```python
from build123d import *

# Parameters (mm, degrees)
SKETCH1_R                     = 14.605
BOSS_EXTRUDE2_DEPTH           = 25.4
SKETCH10_R                    = 5.715
CUT_EXTRUDE5_DEPTH            = 48.424233935
SKETCH11_R                    = 6.6675
CUT_EXTRUDE6_DEPTH            = 1.27
SKETCH12_OUTSIDE_W            = 40.908
SKETCH12_OUTSIDE_H            = 40.908
SKETCH12_OUTSIDE_R            = 10.414
CUT_EXTRUDE7_DEPTH            = 17.78
CIRPATTERN1_COUNT             = 3
CIRPATTERN2_COUNT             = 2
SKETCH26_R                    = 1.651
CUT_EXTRUDE8_DEPTH            = 8.89
CIRPATTERN3_COUNT             = 2
SKETCH27_R                    = 0.79375
CUT_EXTRUDE9_DEPTH            = 24.13
TAP_DRILL_FOR_0_80_TAP3_D     = 1.19126
TAP_DRILL_FOR_0_80_TAP3_DEPTH = 6.35
TAP_DRILL_FOR_0_80_TAP3_TIP   = 0.499792913
TAP_DRILL_FOR_2_56_TAP1_D     = 1.778
CIRPATTERN4_COUNT             = 2


with BuildPart() as part:
    # Sketch1 → Boss-Extrude2 (new body)
    with BuildSketch(Plane(origin=(0, 0, 0), x_dir=(1, 0, 0), z_dir=(0, 1, 0))):
        with Locations(Location((13.028153923, -14.383045271, 0), (0, 0, 270))):
            Circle(SKETCH1_R)
    extrude(amount=BOSS_EXTRUDE2_DEPTH)

    # Sketch10 → Cut-Extrude5 (cut, through all)
    with BuildSketch(Plane(origin=(0, 25.4, 0), x_dir=(1, 0, 0), z_dir=(0, 1, 0))):
        with Locations(Location((13.028153923, -14.383045271, 0), (0, 0, 270))):
            Circle(SKETCH10_R)
    extrude(amount=-CUT_EXTRUDE5_DEPTH, mode=Mode.SUBTRACT)

    # Sketch11 → Cut-Extrude6 (cut)
    with BuildSketch(Plane(origin=(0, 25.4, 0), x_dir=(1, 0, 0), z_dir=(0, 1, 0))):
        with Locations(Location((13.028153923, -14.383045271, 0), (0, 0, 270))):
            Circle(SKETCH11_R)
    extrude(amount=-CUT_EXTRUDE6_DEPTH, mode=Mode.SUBTRACT)

    # Sketch12 outside → Cut-Extrude7 (cut)
    with BuildSketch(Plane(origin=(0, 25.4, 0), x_dir=(1, 0, 0), z_dir=(0, 1, 0))):
        with Locations((13.028, -14.383)):
            Rectangle(SKETCH12_OUTSIDE_W, SKETCH12_OUTSIDE_H)
        with Locations(Location((13.028153923, -14.383045271, 0), (0, 0, 270))):
            Circle(SKETCH12_OUTSIDE_R, mode=Mode.SUBTRACT)
    extrude(amount=-CUT_EXTRUDE7_DEPTH, mode=Mode.SUBTRACT)

    # Sketch17 → #50 (0.07) Diameter Hole1 (revolve, cut)
    with BuildSketch(Plane(origin=(4.692367215, 25.4, 13.504077717), x_dir=(0, 0, 1), z_dir=(1, 0, 0))):
        Polygon((0, 0), (0, 3.07416509), (0.889, 2.54), (0.889, 0), align=None)
    f_50_0_07_diameter_hole1 = revolve(axis=Axis((4.692367215, 31.75, 13.504077717), (0, -1, 0)), mode=Mode.SUBTRACT)

    # CirPattern1: #50 (0.07) Diameter Hole1 ×3 about axis
    cirpattern1_axis = Axis((13.028153923, 0, 14.383045271), (0, 1, 0))
    for i in range(1, CIRPATTERN1_COUNT):
        add(f_50_0_07_diameter_hole1.rotate(cirpattern1_axis, i * 360 / CIRPATTERN1_COUNT), mode=Mode.SUBTRACT)

    # Sketch24 → Tap Drill for #6-32 Tap1 (revolve, cut)
    with BuildSketch(Plane(origin=(8.163266455, 0, 24.388191195), x_dir=(0, 0, -1), z_dir=(1, 0, 0))):
        Polygon((0, 0), (0, 4.81319403), (1.35255, 4.0005), (1.35255, 0), align=None)
    tap_drill_for_6_32_tap1 = revolve(axis=Axis((8.163266455, -6.35, 24.388191195), (0, 1, 0)), mode=Mode.SUBTRACT)

    # CirPattern2: Tap Drill for #6-32 Tap1 ×2 about axis
    cirpattern2_axis = Axis((13.028153923, 0, 14.383045271), (0, 1, 0))
    for i in range(1, CIRPATTERN2_COUNT):
        add(tap_drill_for_6_32_tap1.rotate(cirpattern2_axis, i * 360 / CIRPATTERN2_COUNT), mode=Mode.SUBTRACT)

    # Sketch26 → Cut-Extrude8 (cut)
    with BuildSketch(Plane(origin=(0, 0, 0), x_dir=(-1, 0, 0), z_dir=(0, -1, 0))):
        with Locations(Location((-1.606754466, -8.829520764, 0), (0, 0, 90))):
            Circle(SKETCH26_R)
    cut_extrude8 = extrude(amount=-CUT_EXTRUDE8_DEPTH, mode=Mode.SUBTRACT)

    # CirPattern3: Cut-Extrude8 ×2 about axis
    cirpattern3_axis = Axis((13.028153923, 0, 14.383045271), (0, 1, 0))
    for i in range(1, CIRPATTERN3_COUNT):
        add(cut_extrude8.rotate(cirpattern3_axis, i * 360 / CIRPATTERN3_COUNT), mode=Mode.SUBTRACT)

    # Sketch27 → Cut-Extrude9 (cut)
    with BuildSketch(Plane(origin=(0, 0, 0), x_dir=(-1, 0, 0), z_dir=(0, -1, 0))):
        with Locations(Location((-5.827402564, -17.142659866, 0), (0, 0, 90))):
            Circle(SKETCH27_R)
    extrude(amount=-CUT_EXTRUDE9_DEPTH, mode=Mode.SUBTRACT)

    # Tap Drill for #0-80 Tap3
    with Locations(Plane(origin=(0, 0, 0), x_dir=(-1, 0, 0), z_dir=(0, -1, 0))):
        with Locations((-5.827402564, -15.237659866), (-5.827402564, -19.047659866)):
            Hole(TAP_DRILL_FOR_0_80_TAP3_D / 2, depth=TAP_DRILL_FOR_0_80_TAP3_DEPTH)
            with Locations((0, 0, -(TAP_DRILL_FOR_0_80_TAP3_DEPTH + TAP_DRILL_FOR_0_80_TAP3_TIP / 2))):  # 100° drill point
                Cone(0, TAP_DRILL_FOR_0_80_TAP3_D / 2, TAP_DRILL_FOR_0_80_TAP3_TIP, mode=Mode.SUBTRACT)

    # Tap Drill for #2-56 Tap1 (through all)
    with Locations(Plane(origin=(0.396131886, 0, 13.070787952), x_dir=(0, 0, -1), z_dir=(0, -1, 0))):
        with Locations((0, 0)):
            tap_drill_for_2_56_tap1 = Hole(TAP_DRILL_FOR_2_56_TAP1_D / 2)

    # CirPattern4: Tap Drill for #2-56 Tap1 ×2 about axis
    cirpattern4_axis = Axis((13.028153923, 0, 14.383045271), (0, 1, 0))
    for i in range(1, CIRPATTERN4_COUNT):
        add(tap_drill_for_2_56_tap1.rotate(cirpattern4_axis, i * 360 / CIRPATTERN4_COUNT), mode=Mode.SUBTRACT)


solid = part.part
```
Could you check a few things on this model? Use its own coordinates, in mm. A direction names the side the tool comes from. Give positions to 0.01 mm unless a question says otherwise; leave off trailing zeros. Order: outer loops, then holes, each group sorted by start corner. A loop starts at its lowest first (then second) coordinate and runs counter-clockwise, first axis right, second up.
Q1. Suppose I cut it at B-B, the plane y = 9.75. Write out the boundary of the cut face in (x, z) (1 decimal), and give its area (3 significant figures).
Q2. Suppose I cut it at A-A, the plane x = 10.5. Write out the boundary of the cut face in (y, z).
Q3. I'm going to push flat-ended pins straight in: P1, Ø13, axis at x = 13.03, z = 14.38, coming from the +Y side; P2, Ø12, axis at y = 6, z = 6.5, coming from the -X side; P3, Ø2, axis at x = 1.61, z = 8.83, coming from the +Y side; P4, Ø2, axis at x = 21, y = 20, coming from the -Z side. Where does each tip first touch, or does it pass through?
Q4. For faces 1 (the cylindrical face through (16.89, 12.23, 10.17)), 2 (the cylindrical face through (8.971, 24.774, 9.092)), 3 (the flat face through (6, 24.13, 17)), which set-ups out of +Z, -Z, +X, -X, +Y, -Y let a thin tool reach every point of the face, with its end or its side?
Q5. Suppose I cut it at C-C, the plane x = 14. Write out the boundary of the cut face in (y, z), and give its area (3 significant figures).
Q6. If I drill on line 1 along X through (y, z) = (4.75, 15.5); line 2 along Z through (x, y) = (16, 23); line 3 along Y through (x, z) = (11, 1.5), over which ranges is the centre line in solid material (lowest first)?
Solution:
1. outline: circle Ø20.8 at (13, 14.4); hole circle Ø1.6 at (5.8, 17.1); hole circle Ø11.4 at (13, 14.4)
1. area: 236 mm2
2. outline: (0, 0) - (7.62, 0) - (7.62, 4.28) - (25.4, 4.28) - (25.4, 8.21) - (24.13, 8.21) - (24.13, 9.26) - (0, 9.26) - close; (0, 19.51) - (24.13, 19.51) - (24.13, 20.55) - (25.4, 20.55) - (25.4, 24.49) - (7.62, 24.49) - (7.62, 28.77) - (0, 28.77) - close
3. P1: stops at y = 24.13
3. P2: stops at x = -1.45
3. P3: passes through
3. P4: stops at z = 6.65
4. face 1: +Y, -Y
4. face 2: +Y
4. face 3: -Y
5. outline: (0, -0.19) - (7.62, -0.19) - (7.62, 4.01) - (25.4, 4.01) - (25.4, 7.79) - (24.13, 7.79) - (24.13, 8.75) - (0, 8.75) - close; (0, 20.01) - (24.13, 20.01) - (24.13, 20.98) - (25.4, 20.98) - (25.4, 24.75) - (7.62, 24.75) - (7.62, 28.96) - (0, 28.96) - close
5. area: 302 mm2
6. line 1: x = -1.53 to 5.29, 6.36 to 7.42, 18.63 to 24.79, 26.53 to 27.59
6. line 2: z = 4.4 to 9.5, 19.26 to 21.27, 22.82 to 24.36
6. line 3: y = 0 to 7.62
